```python
from build123d import *

# Parameters (mm, degrees)
SKETCH033_W     = 30
SKETCH033_H     = 32
PAD023_DEPTH    = 6
PAD024_DEPTH    = 6
SKETCH035_R     = 1.6
POCKET011_DEPTH = 6
SKETCH038_W     = 4
SKETCH038_H     = 4
SKETCH038_W_2   = 6
PAD027_DEPTH    = 9
SKETCH039_R     = 1.1
SKETCH039_R_2   = 1
POCKET012_DEPTH = 12
SKETCH040_R     = 10.25
POCKET013_DEPTH = 100
PAD028_DEPTH    = 9
POCKET014_DEPTH = 15
PAD029_DEPTH    = 3
SKETCH043_W     = 12
SKETCH043_H     = 2
POCKET015_DEPTH = 11
SKETCH045_W     = 20
SKETCH045_H     = 6
PAD030_DEPTH    = 20
POCKET016_DEPTH = 12
SKETCH047_R     = 1.6
POCKET017_DEPTH = 6
SKETCH048_R     = 3
POCKET018_DEPTH = 2.5
SKETCH049_R     = 3
POCKET019_DEPTH = 2.5
SKETCH058_R     = 1.05
POCKET021_DEPTH = 8


with BuildPart() as part:
    # Sketch033 → Pad023 (new body)
    with BuildSketch(Plane.XZ):
        Rectangle(SKETCH033_W, SKETCH033_H)
    extrude(amount=PAD023_DEPTH)

    # Sketch034 (on Face6 of Pad023) → Pad024 (join)
    with BuildSketch(Plane.XZ.offset(6)):
        Polygon((-15, 16), (15, 16), (39, 16), (39, -23), (32.5, -23), (32.5, -53), (21.5, -53), (21.5, -23), (17, -23), (17, -16), (15, -16), (-15, -16), (-37, 16), (-37, 32), (-17, 32), (-17, 16), align=None)
    extrude(amount=-PAD024_DEPTH)

    # Sketch035 (on Face14 of Pad024) → Pocket011 (cut)
    with BuildSketch(Plane.XZ.offset(6)):
        with Locations((-10, 10)):
            Circle(SKETCH035_R)
        with Locations((10, 10)):
            Circle(SKETCH035_R)
        with Locations((10, -10)):
            Circle(SKETCH035_R)
        with Locations((-10, -10)):
            Circle(SKETCH035_R)
    extrude(amount=-POCKET011_DEPTH, mode=Mode.SUBTRACT)

    # Sketch038 (on Face5 of Pocket011) → Pad027 (join)
    with BuildSketch(Plane(origin=(0, 0, 0), x_dir=(1, 0, 0), z_dir=(0, 1, 0))):
        with Locations((19, 21)):
            Rectangle(SKETCH038_W, SKETCH038_H)
        with Locations((36, 21)):
            Rectangle(SKETCH038_W_2, SKETCH038_H)
    extrude(amount=PAD027_DEPTH)

    # Sketch039 (on Face21 of Pad027) → Pocket012 (cut)
    with BuildSketch(Plane(origin=(0, 9, 0), x_dir=(1, 0, 0), z_dir=(0, 1, 0))):
        with Locations((19.2, 20.7)):
            Circle(SKETCH039_R)
        with Locations((34.8, 20.7)):
            Circle(SKETCH039_R_2)
    extrude(amount=-POCKET012_DEPTH, mode=Mode.SUBTRACT)

    # Sketch040 (on Face4 of Pocket012) → Pocket013 (cut)
    with BuildSketch(Plane.XZ.offset(6)):
        with Locations((27, 0.5)):
            Circle(SKETCH040_R)
    extrude(amount=-POCKET013_DEPTH, mode=Mode.SUBTRACT)

    # Sketch041 (on Face5 of Pocket013) → Pad028 (join)
    with BuildSketch(Plane(origin=(0, 0, 0), x_dir=(1, 0, 0), z_dir=(0, 1, 0))):
        Polygon((39, -16), (39, 4), (32, 4), (32, 0), (17, 0), (17, -16), align=None)
    extrude(amount=PAD028_DEPTH)

    # Sketch040 (on Face4 of Pocket012) → Pocket014 (cut)
    with BuildSketch(Plane.XZ.offset(6)):
        with Locations((27, 0.5)):
            Circle(SKETCH040_R)
    extrude(amount=-POCKET014_DEPTH, mode=Mode.SUBTRACT)

    # Sketch042 (on Face27 of Pocket014) → Pad029 (join)
    with BuildSketch(Plane(origin=(0, 9, 0), x_dir=(1, 0, 0), z_dir=(0, 1, 0))):
        Polygon((17, -12), (38, -12), (38, 4), (39, 4), (39, -16), (17, -16), align=None)
    extrude(amount=PAD029_DEPTH)

    # Sketch043 (on Face12 of Pad029) → Pocket015 (cut)
    with BuildSketch(Plane(origin=(32.5, 0, 0), x_dir=(0, 0, 1), z_dir=(1, 0, 0))):
        with Locations((-44, 2.5)):
            Rectangle(SKETCH043_W, SKETCH043_H)
    extrude(amount=-POCKET015_DEPTH, mode=Mode.SUBTRACT)

    # Sketch045 (on Face5 of Pocket015) → Pad030 (join)
    with BuildSketch(Plane(origin=(0, 0, 0), x_dir=(1, 0, 0), z_dir=(0, 1, 0))):
        with Locations((-27, -19)):
            Rectangle(SKETCH045_W, SKETCH045_H)
    extrude(amount=PAD030_DEPTH)

    # Sketch046 (on Face26 of Pad030) → Pocket016 (cut)
    with BuildSketch(Plane(origin=(0, 0, 16), x_dir=(1, 0, 0), z_dir=(0, 0, -1))):
        with BuildLine():
            ThreePointArc((-20.7, -10), (-27, -3.7), (-33.3, -10))
            Line((-33.3, -10), (-33.3, -25))
            ThreePointArc((-33.3, -25), (-27, -31.3), (-20.7, -25))
            Line((-20.7, -10), (-20.7, -25))
        make_face()
    extrude(amount=-POCKET016_DEPTH, mode=Mode.SUBTRACT)

    # Sketch047 (on Face4 of Pocket016) → Pocket017 (cut)
    with BuildSketch(Plane.XZ.offset(6)):
        with Locations((10, -4)):
            Circle(SKETCH047_R)
        with Locations((10, 4)):
            Circle(SKETCH047_R)
        with Locations((-10, 0)):
            Circle(SKETCH047_R)
    extrude(amount=-POCKET017_DEPTH, mode=Mode.SUBTRACT)

    # Sketch048 (on Face4 of Pocket017) → Pocket018 (cut)
    with BuildSketch(Plane.XZ.offset(6)):
        with Locations((-10, 10)):
            Circle(SKETCH048_R)
        with Locations((10, 10)):
            Circle(SKETCH048_R)
        with Locations((10, -10)):
            Circle(SKETCH048_R)
        with Locations((-10, -10)):
            Circle(SKETCH048_R)
    extrude(amount=-POCKET018_DEPTH, mode=Mode.SUBTRACT)

    # Sketch049 (on Face5 of Pocket018) → Pocket019 (cut)
    with BuildSketch(Plane(origin=(0, 0, 0), x_dir=(1, 0, 0), z_dir=(0, 1, 0))):
        with Locations((-10, 0)):
            Circle(SKETCH049_R)
        with Locations((10, 4)):
            Circle(SKETCH049_R)
        with Locations((10, -4)):
            Circle(SKETCH049_R)
    extrude(amount=-POCKET019_DEPTH, mode=Mode.SUBTRACT)

    # Sketch058 (on Face50 of Pocket019) → Pocket021 (cut)
    with BuildSketch(Plane(origin=(0, 12, 0), x_dir=(1, 0, 0), z_dir=(0, 1, 0))):
        with Locations((32, -14)):
            Circle(SKETCH058_R)
        with Locations((22, -14)):
            Circle(SKETCH058_R)
    extrude(amount=-POCKET021_DEPTH, mode=Mode.SUBTRACT)


with BuildPart() as part_1:
    # Body005 placement: moved
    add(part.part.moved(Location((-1, -37, 39.4))))


solid = part_1.part
```
CAD build for the part. Positions are in the model's coordinates, mm. A direction names the side the tool comes from. Coordinates: 2 decimals unless noted, no trailing zeros. Write each loop counter-clockwise with the first axis right and the second up, starting at its lowest first coordinate (ties: lowest second). Pieces come first, ordered by that corner, then holes. Notation, with made-up numbers: (-3.5, -19.75) -> (34.5, -19.75) arc R19 ccw to (34.5, -5.75) -> close; hole circle Ø2 at (66, 79). An arc over 180 degrees is marked (long way). Return JSON: item names as keys, results as strings. Group by question number.
Q1. Drill centre lines: line 1 (Z direction, x = -11, y = -37.8); line 2 (Z direction, x = 9, y = -37.8); line 3 (X direction, y = -18.5, z = 61). Where is each one in solid material? Low to high.
Q2. Pull direction X, two halves, no side cores. Call faces 5 (the face through (-38, -33, 60)), 6 (the face through (29, -25, 53)), 7 (the face through (10.3, -40.5, 48.1)): released by +X, released by -X, zero draft, split by the parting line, or undercut.
Q3. Which spindle directions (+Z, -Z, +X, -X, +Y, -Y) get a long thin tool onto all of the face, cutting with end or side? Do faces 1 (the face through (0, -40, 23.4)), 2 (the face through (-9.7, -40.5, 28.1)), 3 (the face through (-28, -34, 61.4)), 4 (the face through (-10, -39.5, 41)). Say none if no direction does.
Q4. Cut at C-C, the plane x = -11. Give the cut face in (y, z).
Q5. Cut at D-D, the plane x = 18.2. Give the cut face in (y, z), then the cut area to 3 significant figures.
Q6. Cut at B-B, the plane z = -1. Give the cut face in (x, y).
Q7. Cut at A-A, the plane x = 26. Give the cut face in (y, z).
Q8. Flat gauge pins, fed straight in: pin 1 (5 mm diameter, centred on x = 9, z = 35.4, fed in from +Y); pin 2 (2.5 mm diameter, centred on x = 21, z = 53.4, fed in from +Y); pin 3 (3.5 mm diameter, centred on x = 27.5, z = -5.5, fed in from +Y). Where does each tip first touch, or does it go through?
Returned:
{
 "1": {"line 1": "z = 23.4 to 27.8, 31 to 36.4, 42.4 to 47.8, 51 to 55.4", "line 2": "z = 23.4 to 27.8, 31 to 32.4, 38.4 to 40.4, 46.4 to 47.8, 51 to 55.4", "line 3": "x = -38 to -34.3, -21.7 to -18"},
 "2": {"face 5": "released by -X", "face 6": "zero draft", "face 7": "undercut"},
 "3": {"face 1": "-Z, -X, +Y, -Y", "face 2": "-Y", "face 3": "+Z, +X, -X, +Y", "face 4": "+Y"},
 "4": {"outline": "(-43, 23.4) -> (-37, 23.4) -> (-37, 27.8) -> (-40.5, 27.8) -> (-40.5, 26.4) -> (-43, 26.4) -> close; (-43, 32.4) -> (-40.5, 32.4) -> (-40.5, 31) -> (-37, 31) -> (-37, 36.4) -> (-39.5, 36.4) -> (-39.5, 37.8) -> (-43, 37.8) -> close; (-43, 41) -> (-39.5, 41) -> (-39.5, 42.4) -> (-37, 42.4) -> (-37, 47.8) -> (-40.5, 47.8) -> (-40.5, 46.4) -> (-43, 46.4) -> close; (-43, 52.4) -> (-40.5, 52.4) -> (-40.5, 51) -> (-37, 51) -> (-37, 55.4) -> (-43, 55.4) -> close"},
 "5": {"outline": "(-43, 16.4) -> (-28, 16.4) -> (-28, 17.6) -> (-40, 17.6) -> (-40, 19.8) -> (-28, 19.8) -> (-28, 20.4) -> (-37, 20.4) -> (-37, 33.25) -> (-43, 33.25) -> close; (-43, 46.55) -> (-28, 46.55) -> (-28, 51.4) -> (-25, 51.4) -> (-25, 55.4) -> (-43, 55.4) -> close", "area": "255 mm2"},
 "6": {"outline": "(20.5, -43) -> (31.5, -43) -> (31.5, -40.5) -> (20.5, -40.5) -> close; (20.5, -38.5) -> (31.5, -38.5) -> (31.5, -37) -> (20.5, -37) -> close"},
 "7": {"outline": "(-43, -13.6) -> (-37, -13.6) -> (-37, 29.65) -> (-43, 29.65) -> close; (-43, 50.15) -> (-28, 50.15) -> (-28, 51.4) -> (-25, 51.4) -> (-25, 55.4) -> (-43, 55.4) -> close; hole (-40.5, -10.6) -> (-38.5, -10.6) -> (-38.5, 1.4) -> (-40.5, 1.4) -> close"},
 "8": {"pin 1": "stops at y = -39.5", "pin 2": "stops at y = -25", "pin 3": "stops at y = -37"}
}
